from build123d import *


with BuildPart() as part:
    # Эскиз1 → Повернуть1 (revolve)
    with BuildSketch(Plane.XY, mode=Mode.PRIVATE) as revolve_1_sk:
        with BuildLine():
            Line((1.1, 1), (2, 1))
            ThreePointArc((2, 1), (3.118033989, 0.736067977), (4, 0))
            Line((4, 0), (2, 0))
            Line((2, 0), (2, -5))
            ThreePointArc((2, -5), (3, -6), (2, -7))
            Line((2, -7), (1.1, -7))
            Line((1.1, -7), (1.1, 1))
        make_face()
    revolve(revolve_1_sk.sketch.rotate(Axis((0, -12.837811583, 0), (0, 1, 0)), 90), axis=Axis((0, -12.837811583, 0), (0, 1, 0)))


solid = part.part
Design review of the part built by this model. Coordinates are the model's own, in mm. A direction names the side the tool comes from. Coordinates: 2 decimals unless noted, no trailing zeros. Write each loop counter-clockwise with the first axis right and the second up, starting at its lowest first coordinate (ties: lowest second). Pieces come first, ordered by that corner, then holes. Notation, with made-up numbers: (9, 23.5) -> (47, 23.5) arc R8 cw to (47, 30.5) -> close; hole circle Ø5 at (3.25, -39). An arc over 180 degrees is marked (long way). Write each question's results on one line, items separated by ' | '. Start each with the question number.
(1) Clearance check with flat-ended pins moving along their axes: P1, Ø2, axis at y = -5, z = 0.5, coming from the -X side; P2, Ø3, axis at x = 3, y = -4, coming from the +Z side; P3, Ø4, axis at y = -2.5, z = -2, coming from the -X side. State where each tip first meets the part, or that it passes through.
(2) Take a section at A-A on y = -2.75. Write out the cut boundary in (x, z), and give its area (3 significant figures).
(3) Tool access review of faces 1 (the face through (1, 0, 2)), 2 (the face through (1, 1, 1)): name each direction out of +Z, -Z, +X, -X, +Y, -Y from which nothing blocks a thin tool from reaching the whole face with its end or side.
(4) The part is to be moulded in two halves that separate along X. For faces 3 (the face through (2, -3, 0)), 4 (the face through (1, -7, -1)), 5 (the face through (-1.09, -2.94, 0.14)), say which applies: pulls with the +X half, pulls with the -X half, needs draft (parallel to the pull), parting line crosses it, or undercut.
(5) For line 1 along X through (y, z) = (-3.75, 0); line 2 along X through (y, z) = (-6.5, -1); line 3 along Z through (x, y) = (0.75, -1), list the stretches that pass through material, from the lowest coordinate up. Write a range as from..to.
Results found:
1) P1: stops at x = -2.99 | P2: stops at z = 1.54 | P3: stops at x = -2
2) outline: circle Ø4 at (0, 0); hole circle Ø2.2 at (0, 0) | area: 8.77 mm2
3) face 1: none | face 2: +Z, -Z, +X, -X, +Y
4) face 3: parting line crosses it | face 4: needs draft | face 5: undercut
5) line 1: x = -2..-1.1, 1.1..2 | line 2: x = -2.69..-0.46, 0.46..2.69 | line 3: z = -1.85..-0.8, 0.8..1.85
